The listing builds one solid part. Answer for the finished solid, in the listing's coordinates (mm). Round coordinates to 2 decimals unless told otherwise and drop trailing zeros. Loops run counter-clockwise (first coordinate to the right, second up) from the corner with the lowest first, then second, coordinate; pieces in that order, holes last. Notation, with made-up numbers: (70, 52.25) -> (97, 52.25) arc R11 cw to (97, 59.25) -> close; hole circle Ø7 at (71, 75). An arc over 180 degrees is marked (long way). Use a Markdown table: item, result. Add a question column.
Q1. Consider line 1 (Y direction, x = 3.3, z = -24.14); line 2 (Y direction, x = 2.85, z = 24.14); line 3 (Z direction, x = 3.9, y = -20). Determine where each line is inside the solid, lowest interval first.
Q2. Section A-A on z = 24.14 is taken. Give the vertices of the cut face in (x, y), then the cut area to 3 significant figures.
Q3. For a pull along Z with two mould halves and no side action, classify faces 1 (the flat face through (4.5, 1, 1)), 2 (the cylindrical face through (2.22, -25.66, -22.64)), 3 (the flat face through (2, -1, 40)) as released by +Z, released by -Z, zero draft, split by the parting line, or undercut.
Q4. Given pin 1 Ø1.9 at (y, z) = (-18.7, 24.14) entering from -X, flat-ended and moving along its own axis, determine where the tip first touches the part or whether it passes through.
Q5. Section B-B on y = -18.7 is taken. Give the vertices of the cut face in (x, z), then the cut area to 3 significant figures.
Q6. Section C-C on z = -24.12 is taken. Give the vertices of the cut face in (x, y).
from build123d import *

# Parameters (mm, degrees)
SKETCH1_W           = 80
SKETCH1_H           = 160
BOSS_EXTRUDE1_DEPTH = 4.5
SKETCH2_R           = 1.6
CUT_EXTRUDE1_DEPTH  = 4.5


with BuildPart() as part:
    # Sketch1 → Boss-Extrude1 (new body)
    with BuildSketch(Plane(origin=(0, 0, 0), x_dir=(0, 0, -1), z_dir=(1, 0, 0))):
        Rectangle(SKETCH1_W, SKETCH1_H)
    extrude(amount=BOSS_EXTRUDE1_DEPTH)

    # Sketch2 → Cut-Extrude1 (cut)
    with BuildSketch(Plane.ZY):
        with Locations((-24.14, 57.5)):
            Circle(SKETCH2_R)
        with Locations((24.14, 56.23)):
            Circle(SKETCH2_R)
        with Locations((24.14, -18.7)):
            Circle(SKETCH2_R)
        with Locations((-24.12, -25.05)):
            Circle(SKETCH2_R)
    extrude(amount=-CUT_EXTRUDE1_DEPTH, mode=Mode.SUBTRACT)


solid = part.part
Checked values:
| question | item | result |
|---|---|---|
| 1 | line 1 | y = -80 to -26.65, -23.45 to 55.9, 59.1 to 80 |
| 1 | line 2 | y = -80 to -20.3, -17.1 to 54.63, 57.83 to 80 |
| 1 | line 3 | z = -40 to 23.21, 25.07 to 40 |
| 2 | outline | (0, -80) -> (4.5, -80) -> (4.5, -20.3) -> (0, -20.3) -> close; (0, -17.1) -> (4.5, -17.1) -> (4.5, 54.63) -> (0, 54.63) -> close; (0, 57.83) -> (4.5, 57.83) -> (4.5, 80) -> (0, 80) -> close |
| 2 | area | 691 mm2 |
| 3 | face 1 | zero draft |
| 3 | face 2 | undercut |
| 3 | face 3 | released by +Z |
| 4 | pin 1 | passes through |
| 5 | outline | (0, -40) -> (4.5, -40) -> (4.5, 22.54) -> (0, 22.54) -> close; (0, 25.74) -> (4.5, 25.74) -> (4.5, 40) -> (0, 40) -> close |
| 5 | area | 346 mm2 |
| 6 | outline | (0, -80) -> (4.5, -80) -> (4.5, -26.65) -> (0, -26.65) -> close; (0, -23.45) -> (4.5, -23.45) -> (4.5, 55.9) -> (0, 55.9) -> close; (0, 59.1) -> (4.5, 59.1) -> (4.5, 80) -> (0, 80) -> close |
